Drawing for the job (mm, zero at the part's lowest x, y, z). A direction names the side the tool comes from. Coordinates: 2 decimals unless noted, no trailing zeros. Write each loop counter-clockwise with the first axis right and the second up, starting at its lowest first coordinate (ties: lowest second). Pieces come first, ordered by that corner, then holes. Notation, with made-up numbers: (63, 17) - (118, 17) arc R32 ccw to (118, 56) - close; hole circle Ø2 at (9.5, -19.75). An arc over 180 degrees is marked (long way). Write each question's results on one line, items separated by ' | '.
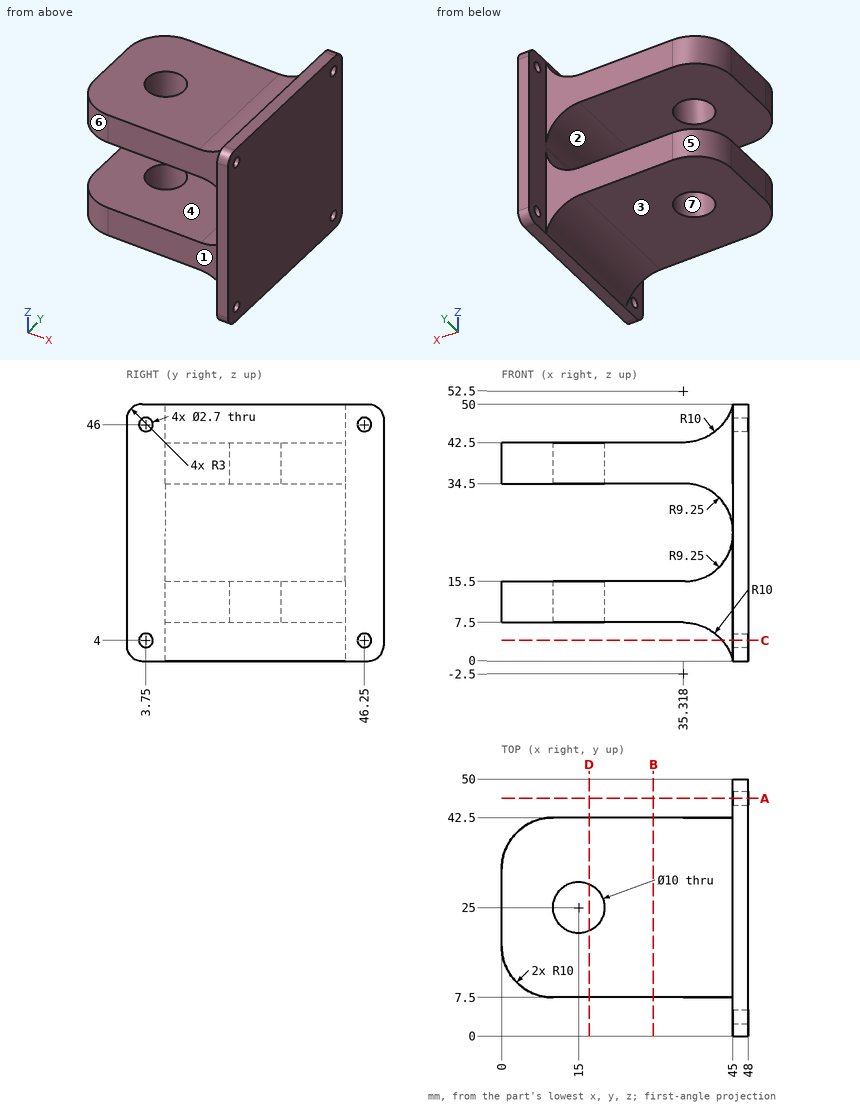
(1) Wall check: line 1 (Y direction, x = 46.5, z = 46); line 2 (Z direction, x = 23, y = 41); line 3 (Z direction, x = 47, y = 46). Give the ranges that are in metal, low to high. Write a range as from..to.
Return value:
line 1: y = 0..2.4, 5.1..44.9, 47.6..50 | line 2: z = 7.5..15.5, 34.5..42.5 | line 3: z = 0..2.67, 5.33..44.67, 47.33..50
(2) Flat gauge pins, fed straight in: P1, Ø12.5, axis at x = 21, z = 34, coming from the -Y side; P2, Ø1.5, axis at x = 36.5, z = 41.5, coming from the +Y side; P3, Ø6, axis at x = 30.5, y = 13.5, coming from the +Z side. Where does each tip first touch, or does it go through?
Return value:
P1: stops at y = 7.5 | P2: stops at y = 42.5 | P3: stops at z = 42.5
(3) Saw through at C-C on z = 4. Write the cut outline in (x, y), then the cut area to 3 significant figures.
Return value:
outline: (42.92, 7.5) - (45, 7.5) - (45, 5.1) - (48, 5.1) - (48, 44.9) - (45, 44.9) - (45, 42.5) - (42.92, 42.5) - close; (45, 0) - (48, 0) - (48, 2.4) - (45, 2.4) - close; (45, 47.6) - (48, 47.6) - (48, 50) - (45, 50) - close | area: 207 mm^2
(4) Saw through at B-B on x = 29.5. Write the cut outline in (y, z), then the cut area to 3 significant figures.
Return value:
outline: (7.5, 7.5) - (42.5, 7.5) - (42.5, 15.5) - (7.5, 15.5) - close; (7.5, 34.5) - (42.5, 34.5) - (42.5, 42.5) - (7.5, 42.5) - close | area: 560 mm^2
(5) Saw through at D-D on x = 17. Write the cut outline in (y, z).
Return value:
outline: (7.5, 7.5) - (20.42, 7.5) - (20.42, 15.5) - (7.5, 15.5) - close; (7.5, 34.5) - (20.42, 34.5) - (20.42, 42.5) - (7.5, 42.5) - close; (29.58, 7.5) - (42.5, 7.5) - (42.5, 15.5) - (29.58, 15.5) - close; (29.58, 34.5) - (42.5, 34.5) - (42.5, 42.5) - (29.58, 42.5) - close
(6) 3-axis set-ups, long thin cutter, end or side, ignore diameter. For the marked faces 1, 2 and 3: which of +Z, -Z, +X, -X, +Y, -Y reach the whole face in a straight line?
Return value:
face 1: +Z, -Z, -X, -Y | face 2: -X, +Y, -Y | face 3: -Z, -X, +Y, -Y
(7) Saw through at A-A on y = 46.25. Write the cut outline in (x, z).
Return value:
outline: (45, 0) - (48, 0) - (48, 2.65) - (45, 2.65) - close; (45, 5.35) - (48, 5.35) - (48, 44.65) - (45, 44.65) - close; (45, 47.35) - (48, 47.35) - (48, 50) - (45, 50) - close
(8) Two-plate mould, pull along Y, no slides. Class the marked faces 4, 5, 6 and 7: released by +Y, released by -Y, zero draft, split by the parting line, or undercut.
Return value:
face 4: zero draft | face 5: released by +Y | face 6: released by -Y | face 7: undercut
